Model file for the job. Use its own axes, mm. Coordinates: 2 decimals unless noted, no trailing zeros. Write each loop counter-clockwise with the first axis right and the second up, starting at its lowest first coordinate (ties: lowest second). Pieces come first, ordered by that corner, then holes.
Q1. Drill centre lines: probe 1 along Y at (x, z) = (2.85, 443.5); probe 2 along Y at (x, z) = (3.45, 245.5); probe 3 along Z at (x, y) = (1.9, 116.5). Where is each one in solid material? Low to high.
Q2. Band-saw the part on C-C, the plane x = 1.7. State how many separate pieces and enclosed holes the cut face has, plus the area to 3 significant figures.
Q3. Band-saw the part on D-D, the plane y = -44. Write the cut outline in (x, z), plus the area to 3 significant figures.
Q4. Band-saw the part on A-A, the plane y = 121.5. Write the cut outline in (x, z).
Q5. Band-saw the part on B-B, the plane z = 174. Write the cut outline in (x, y).
Q6. Pull direction Z, two halves, no side cores. Call faces 1 (the cylindrical face through (2.83, 67.8, 217.03)), 2 (the cylindrical face through (2.755, -115.083, 430.712)), 3 (the cylindrical face through (2.75, -14.36, 481.82)): released by +Z, released by -Z, zero draft, split by the parting line, or undercut.
Q7. Pin check, flat tips, straight feed: P1, Ø1, axis at x = 3.5, y = -26, coming from the +Z side; P2, Ø17, axis at y = 49.31, z = 368.15, coming from the +X side; P3, Ø3, axis at x = 1.5, z = 56.5, coming from the -Y side. Stop position of each tip, or through.
from build123d import *

# Parameters (mm, degrees)
SKETCH2_R           = 14.2875
SKETCH2_R_2         = 19.05
SKETCH2_R_3         = 2.5527
SKETCH2_R_4         = 5.0419
SKETCH2_R_5         = 3.3782
SKETCH2_R_6         = 5.08
BOSS_EXTRUDE1_DEPTH = 5.588
SKETCH4_R           = 31.75
SKETCH4_R_2         = 2.54
CUT_EXTRUDE1_DEPTH  = 6.588


with BuildPart() as part:
    # Sketch2 → Boss-Extrude1 (new body)
    with BuildSketch(Plane(origin=(0, 0, 0), x_dir=(0, 0, -1), z_dir=(1, 0, 0))):
        with BuildLine():
            Line((-456.118369633, -95.925064686), (-472.468769944, -31.298651711))
            ThreePointArc((-472.468769944, -31.298651711), (-482.016027605, -14.158478394), (-498.826247655, -4.041553364))
            ThreePointArc((-498.826247655, -4.041553364), (-507.892088549, 6.507023908), (-501.854140922, 19.037193183))
            Line((-501.854140922, 19.037193183), (-398.295274803, 81.43217891))
            ThreePointArc((-398.295274803, 81.43217891), (-397.645900343, 81.797901654), (-396.976191421, 82.124903604))
            Line((-396.976191421, 82.124903604), (-287.837435211, 131.503170214))
            ThreePointArc((-287.837435211, 131.503170214), (-276.093947879, 138.70177912), (-266.497227284, 148.582690958))
            Line((-266.497227284, 148.582690958), (-253.809934756, 165.419296806))
            ThreePointArc((-253.809934756, 165.419296806), (-244.745753976, 170.430370198), (-234.964294435, 167.025479743))
            Line((-234.964294435, 167.025479743), (-208.040592879, 141.691905515))
            ThreePointArc((-208.040592879, 141.691905515), (-202.97415121, 137.465830921), (-197.439882679, 133.87411692))
            Line((-197.439882679, 133.87411692), (9.397681692, 16.570639059))
            ThreePointArc((9.397681692, 16.570639059), (17.93346767, -6.425981428), (-3.265021391, -18.768114858))
            Line((-3.265021391, -18.768114858), (-232.00028645, 21.024135937))
            ThreePointArc((-232.00028645, 21.024135937), (-342.59010045, -2.271898683), (-406.726541812, -95.327414797))
            ThreePointArc((-406.726541812, -95.327414797), (-431.186900503, -115.093327518), (-456.118369633, -95.925064686))
        make_face()
        with Locations((-236.525067803, 126.839996455)):
            Circle(SKETCH2_R, mode=Mode.SUBTRACT)
        with Locations((-368.146285671, 49.309174015)):
            Circle(SKETCH2_R, mode=Mode.SUBTRACT)
        with Locations((-431.494222517, -89.695186775)):
            Circle(SKETCH2_R, mode=Mode.SUBTRACT)
        with Locations((-450.85, 12.7)):
            Circle(SKETCH2_R_2, mode=Mode.SUBTRACT)
        with Locations((-344.900370281, 26.063258625)):
            Circle(SKETCH2_R_3, mode=Mode.SUBTRACT)
        Circle(SKETCH2_R_4, mode=Mode.SUBTRACT)
        with Locations((-71.568668283, 6.261447138)):
            Circle(SKETCH2_R_5, mode=Mode.SUBTRACT)
        with Locations((-391.74113388, 70.554070767)):
            Circle(SKETCH2_R_5, mode=Mode.SUBTRACT)
        with Locations((-243.667263779, 157.776246012)):
            Circle(SKETCH2_R_5, mode=Mode.SUBTRACT)
        with Locations((-432.889487758, 30.660512242)):
            Circle(SKETCH2_R_6, mode=Mode.SUBTRACT)
        with Locations((-468.810512242, 30.660512242)):
            Circle(SKETCH2_R_3, mode=Mode.SUBTRACT)
        with Locations((-468.810512242, -5.260512242)):
            Circle(SKETCH2_R_6, mode=Mode.SUBTRACT)
        with Locations((-432.889487758, -5.260512242)):
            Circle(SKETCH2_R_3, mode=Mode.SUBTRACT)
        with Locations((-495.3, 8.15908504)):
            Circle(SKETCH2_R_5, mode=Mode.SUBTRACT)
    extrude(amount=BOSS_EXTRUDE1_DEPTH)

    # Sketch4 → Cut-Extrude1 (cut, through all)
    with BuildSketch(Plane(origin=(5.588, 0, 0), x_dir=(0, 0, -1), z_dir=(1, 0, 0))):
        with Locations((-294.8848929, 71.606423498)):
            Circle(SKETCH4_R)
        with Locations((-185.31249926, 66.401808093)):
            Circle(SKETCH4_R)
        with Locations((-316.523268338, 111.55499619)):
            Circle(SKETCH4_R_2)
        with Locations((-161.782656077, 106.351776712)):
            Circle(SKETCH4_R_2)
        with Locations((-77.758767474, 58.699434709)):
            Circle(SKETCH4_R_2)
    extrude(amount=-CUT_EXTRUDE1_DEPTH, mode=Mode.SUBTRACT)


solid = part.part
Answer sheet:
1. probe 1: y = -112.08 to -97.44, -81.95 to -4.87, 30.27 to 54.2
1. probe 2: y = 22.76 to 115.72, 137.96 to 154.94, 160.61 to 170.34
1. probe 3: z = 166.8 to 226.67, 246.38 to 321
2. separate pieces: 1
2. enclosed holes: 19
2. area: 43,900 mm2
3. outline: (0, 384.53) - (5.59, 384.53) - (5.59, 469.26) - (0, 469.26) - close
3. area: 473 mm2
4. outline: (0, 175.62) - (5.59, 175.62) - (5.59, 223.27) - (0, 223.27) - close; (0, 249.78) - (5.59, 249.78) - (5.59, 309.95) - (0, 309.95) - close
5. outline: (0, 10.93) - (5.59, 10.93) - (5.59, 36.74) - (0, 36.74) - close; (0, 96.07) - (5.59, 96.07) - (5.59, 120.58) - (0, 120.58) - close
6. face 1: undercut
6. face 2: split by the parting line
6. face 3: released by +Z
7. P1: stops at z = 474.44
7. P2: passes through
7. P3: stops at y = -9.77
